Could you check a few things on this model? Use its own coordinates, in mm. A direction names the side the tool comes from. Give positions to 0.01 mm unless a question says otherwise; leave off trailing zeros. Write each loop counter-clockwise with the first axis right and the second up, starting at its lowest first coordinate (ties: lowest second). Pieces come first, ordered by that corner, then holes. Notation, with made-up numbers: (73, 29.5) - (85, 29.5) arc R16 cw to (85, 36.5) - close; hole circle Ø6 at (-19, -8). An arc over 180 degrees is marked (long way). Answer in a Markdown table with one row per item.
from build123d import *

# Parameters (mm, degrees)
F1_DEPTH = 30
F3_DEPTH = 40
F5_DEPTH = 70
F7_DEPTH = 130.001


with BuildPart() as f1:
    # F0 (on Front) → F1 (new body)
    with BuildSketch(Plane.XZ):
        Polygon((35, -45), (35, 65), (-35, 65), (-35, -45), (-35, -65), (-15, -65), (-15, -45), (15, -45), (15, -65), (35, -65), align=None)
    extrude(amount=F1_DEPTH)

    # F2 (on face) → F3 (join)
    with BuildSketch(Plane.XZ.offset(30)):
        Polygon((-20, 65), (-35, 65), (-35, 50), (-35, 30), (-35, 15), (-20, 15), (20, 15), (35, 15), (35, 30), (35, 50), (35, 65), (20, 65), align=None)
    extrude(amount=F3_DEPTH)

    # F4 (on face) → F5 (join)
    with BuildSketch(Plane.YZ.offset(35)):
        Polygon((-70, 15), (-30, -25), (-30, 15), align=None)
    extrude(amount=-F5_DEPTH)

    # F6 (on face) → F7 (cut, through all)
    with BuildSketch(Plane.XY.offset(65)):
        with BuildLine():
            Line((15, -45), (-15, -45))
            ThreePointArc((-15, -45), (-18.535534, -46.464466), (-20, -50))
            Line((-20, -50), (-20, -60))
            ThreePointArc((-20, -60), (-18.535534, -63.535534), (-15, -65))
            Line((-15, -65), (15, -65))
            ThreePointArc((15, -65), (18.535534, -63.535534), (20, -60))
            Line((20, -60), (20, -50))
            ThreePointArc((20, -50), (18.535534, -46.464466), (15, -45))
        make_face()
    extrude(amount=-F7_DEPTH, mode=Mode.SUBTRACT)


solid = f1.part
1) Imagine slicing it at D-D (z = -54). List the corners of the cut face in (x, y) for me, then the cut area to 3 significant figures.
Check values:
| item | result |
|---|---|
| outline | (-35, -30) - (-15, -30) - (-15, 0) - (-35, 0) - close; (15, -30) - (35, -30) - (35, 0) - (15, 0) - close |
| area | 1,200 mm2 |
2) We'd pull the mould along Y, two halves only. Please class faces 1 (the face through (0, -15, -45)), 2 (the face through (0, -65, 38)), 3 (the face through (-0.5, -30, -44.7)): +Y half, -Y half, draft (parallel to the pull), parting line (faces both ways), or undercut.
Check values:
| item | result |
|---|---|
| face 1 | draft |
| face 2 | undercut |
| face 3 | -Y half |
3) Imagine slicing it at A-A (x = 0). List the corners of the cut face in (y, z) for me, then the cut area to 3 significant figures.
Check values:
| item | result |
|---|---|
| outline | (-70, 15) - (-65, 10) - (-65, 65) - (-70, 65) - close; (-45, -10) - (-30, -25) - (-30, -45) - (0, -45) - (0, 65) - (-45, 65) - close |
| area | 4,800 mm2 |
4) Imagine slicing it at C-C (z = 42.5). List the corners of the cut face in (x, y) for me.
Check values:
| item | result |
|---|---|
| outline | (-35, -70) - (35, -70) - (35, 0) - (-35, 0) - close; hole (-20, -60) arc R5 ccw to (-15, -65) - (15, -65) arc R5 ccw to (20, -60) - (20, -50) arc R5 ccw to (15, -45) - (-15, -45) arc R5 ccw to (-20, -50) - close |
5) Will these pins go through, and if not, where does the flat tip stop? P1, Ø4, axis at x = 18.5, z = 8, coming from the +Y side; P2, Ø24, axis at x = -2, y = -17, coming from the -Z side.
Check values:
| item | result |
|---|---|
| P1 | stops at y = 0 |
| P2 | stops at z = -45 |
6) Imagine slicing it at B-B (y = -52). List the corners of the cut face in (x, z) for me.
Check values:
| item | result |
|---|---|
| outline | (-35, -3) - (-20, -3) - (-20, 65) - (-35, 65) - close; (20, -3) - (35, -3) - (35, 65) - (20, 65) - close |
7) On a 3-axis mill with a long thin cutter (end or side, diameter ignored), from which of +Z, -Z, +X, -X, +Y, -Y can I reach the whole of each face in a straight line? I mean faces 4 (the face through (-15, -15, -55)), 5 (the face through (-25, -15, -65)), 6 (the face through (20, -55, 30)). Say none if no direction works.
Check values:
| item | result |
|---|---|
| face 4 | -Z, +Y, -Y |
| face 5 | -Z, +X, -X, +Y, -Y |
| face 6 | +Z, -Z |
8) If I drill on line 1 (X direction, y = -58, z = 46); line 2 (X direction, y = -24.5, z = -57); line 3 (Y direction, x = -1.5, z = 35), over which ranges is the centre line in solid material (lowest first)?
Check values:
| item | result |
|---|---|
| line 1 | x = -35 to -20, 20 to 35 |
| line 2 | x = -35 to -15, 15 to 35 |
| line 3 | y = -70 to -65, -45 to 0 |
